```python
from build123d import *

# Parameters (mm, degrees)
SKETCH2_R = 8.35


with BuildPart() as part:
    # Sweep1: sweep along a path in Sketch1
    with BuildLine(Plane(origin=(0, 0, 0), x_dir=(1, 0, 0), z_dir=(0, 1, 0))) as sweep1_path:
        Line((-260.025, 0), (-260.025, -95))
        ThreePointArc((-260.025, -95), (-248.309271247, -123.284271247), (-220.025, -135))
        Line((-220.025, -135), (220.025, -135))
        ThreePointArc((220.025, -135), (248.309271247, -123.284271247), (260.025, -95))
        Line((260.025, -95), (260.025, 0))
    # Sketch2 → Sweep1 (sweep)
    with BuildSketch(Plane.XY):
        with Locations((260.025, 0)):
            Circle(SKETCH2_R)
    sweep(path=sweep1_path.line)


solid = part.part
```
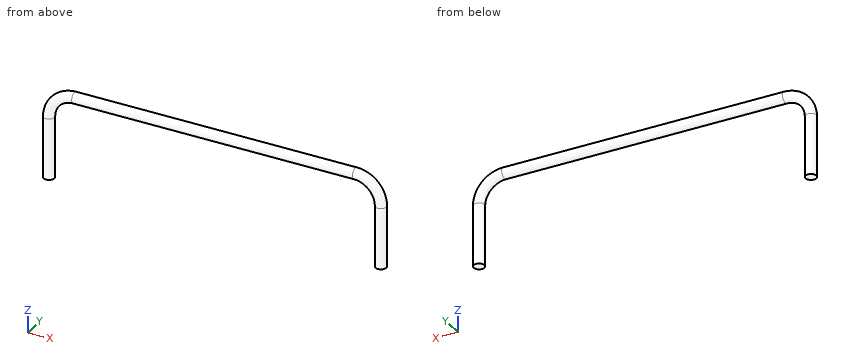
Geometry: final body of the model. Coordinates: model frame, mm. Coordinates: 2 decimals unless noted, no trailing zeros. Write each loop counter-clockwise with the first axis right and the second up, starting at its lowest first coordinate (ties: lowest second). Pieces come first, ordered by that corner, then holes. Notation, with made-up numbers: M 53,-23.75 L 104,-23.75 A24 ccw 104,2.25 Z; hole C 52,10 d9. An arc over 180 degrees is marked long. Answer as CSV lines item,"result". Start each with the question number.
Q1. Cut plane A-A on z = 60.5. Return the cut outline in (x, y) (3 decimals).
Q2. Cut plane C-C on x = 29.5. Return the cut outline in (y, z), then the cut area to 3 significant figures.
Q3. Pin query (flat end, axial travel): P1, Ø5, axis at x = 110, y = -4.5, coming from the +Z side; P2, Ø1, axis at x = -190, y = 1, coming from the -Z side (3 decimals); P3, Ø4, axis at x = -194.5, y = -4, coming from the -Z side. Return the tip coordinate at first contact, or that it passes through.
Q4. Cut plane B-B on y = 0. Return the cut outline in (x, z) (3 decimals), then the cut area to 3 significant figures.
Q5. Line query: line 1 (X direction, y = -0.25, z = 58.5); line 2 (Z direction, x = 20, y = 1.25); line 3 (X direction, y = 3.75, z = 77.5). Output: solid intervals per line, ascending. Write a range as from..to.
Findings below:
1,outline,"C -260.025,0 d16.7; C 260.025,0 d16.7"
2,outline,"C 0,135 d16.7"
2,area,"219 mm2"
3,P1,"stops at z = 143.11"
3,P2,"stops at z = 126.665"
3,P3,"stops at z = 126.89"
4,outline,"M -268.375,0 L -251.675,0 L -251.675,95 A31.65 cw -220.025,126.65 L 220.025,126.65 A31.65 cw 251.675,95 L 251.675,0 L 268.375,0 L 268.375,95 A48.35 ccw 220.025,143.35 L -220.025,143.35 A48.35 ccw -268.375,95 Z"
4,area,"12,600 mm2"
5,line 1,"x = -268.37..-251.68, 251.68..268.37"
5,line 2,"z = 126.74..143.26"
5,line 3,"x = -267.49..-252.56, 252.56..267.49"
